from build123d import *

# Parameters (mm, degrees)
F1_DEPTH = 36
F2_R     = 70
F3_SIZE  = 12


with BuildPart() as f1:
    # F0 (on Front) → F1 (new body)
    with BuildSketch(Plane.XZ):
        Polygon((-119.609225, 1.666667), (-45, -158.333333), (45, -158.333333), (119.609225, 1.666667), (200, 1.666667), (200, 61.666667), (-200, 61.666667), (-200, 1.666667), align=None)
    extrude(amount=F1_DEPTH)

    # F2
    f2_edges = [f1.edges().sort_by_distance(p)[0] for p in [
        (119.609225, -18, 1.666667),
        (-119.609225, -18, 1.666667),
    ]]
    fillet(f2_edges, radius=F2_R)

    # F3
    f3_edges = [f1.edges().sort_by_distance(p)[0] for p in [
        (0, -36, 61.666667),
        (182.102072, -36, 1.666667),
        (-72.881299, -36, -98.541694),
        (0, -36, -158.333333),
    ]]
    chamfer(f3_edges, length=F3_SIZE)


solid = f1.part
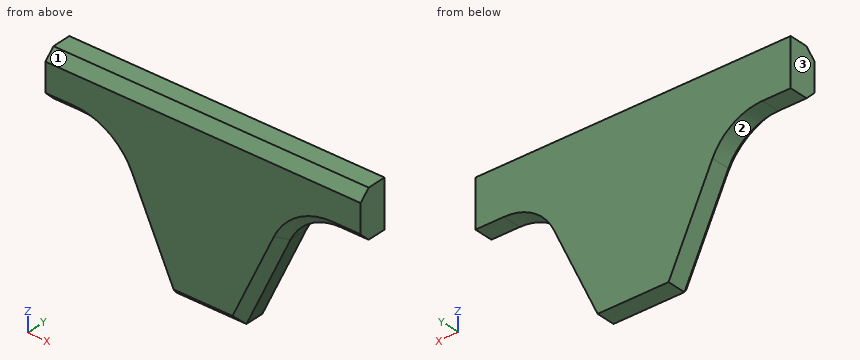
Input: part model. Units: mm. Frame: model coordinates. Face numbers are marked on the shaded views. Give positions to 0.01 mm unless a question says otherwise; leave off trailing zeros. Write each loop counter-clockwise with the first axis right and the second up, starting at its lowest first coordinate (ties: lowest second). Pieces come first, ordered by that corner, then holes. Notation, with made-up numbers: M -31.75,-32.75 L 3.25,-32.75 A24 cw 3.25,-21.75 Z; hole C -20,-21 d5. An arc over 180 degrees is marked long. Use one line per item in the form item = value.
1. Cut plane A-A on y = -15.5. Return loops of the section in (x, z).
Outcome:
outline = M -200,1.67 L -164.2,1.67 A70 cw -100.76,-38.75 L -45,-158.33 L 45,-158.33 L 100.76,-38.75 A70 cw 164.2,1.67 L 200,1.67 L 200,61.67 L -200,61.67 Z
2. First-contact query: P1, Ø12, axis at y = -7.5, z = -118.5, coming from the -X side; P2, Ø19, axis at x = -179, y = -11.5, coming from the -Z side; P3, Ø6, axis at y = -23, z = -51.5, coming from the +X side. Flat tips, straight axial feed; report the tip coordinate or a pass-through.
Outcome:
P1 = -66.37
P2 = 1.67
P3 = 96.22
3. Cut plane B-B on z = -66.5. Return loops of the section in (x, y), and give its area (3 significant figures).
Outcome:
outline = M -87.82,-24 L -74.58,-36 L 74.58,-36 L 87.82,-24 L 87.82,0 L -87.82,0 Z
area = 6,160 mm²
4. Cut plane C-C on z = -101.5. Return loops of the section in (x, y), and give its area (3 significant figures).
Outcome:
outline = M -71.5,-24 L -58.26,-36 L 58.26,-36 L 71.5,-24 L 71.5,0 L -71.5,0 Z
area = 4,990 mm²
5. Ray query, L1, parallel to Y at x = -41.5, z = 52; L2, parallel to X at y = -10, z = -111; L3, parallel to Z at x = 97, y = -4. Return the intervals inside material, ascending.
Outcome:
L1 = -33.67 to 0
L2 = -67.07 to 67.07
L3 = -46.82 to 61.67
6. Mould query, pull axis Z, two halves, no side actions, for the marked faces 1, 2 and 3. Classes: released by +Z, released by -Z, zero draft, split by the parting line, or undercut.
Outcome:
face_1 = released by +Z
face_2 = released by -Z
face_3 = zero draft
